Autodesk Inventor part; units mm, degrees
ref_plane "YZ Plane" through (0, 0, 0) normal (1, 0, 0) x (0, 1, 0)
ref_plane "XZ Plane" through (0, 0, 0) normal (0, 1, 0) x (-1, 0, 0)
ref_plane "XY Plane" through (0, 0, 0) normal (0, 0, 1) x (1, 0, 0)
sketch "Sketch1" plane through (0, 0, 0) normal (0, 0, 1) x (1, 0, 0)
  line L0 (0, 0) -> (9.525, 0)
  line L1 (9.525, 0) -> (9.525, 25.4)
  line L2 (9.525, 25.4) -> (0, 25.4)
  line L3 (0, 25.4) -> (0, 0)
  dimension "d0" = 9.525
  dimension "d1" = 25.4
extrude "Extrusion1" add sketch "Sketch1" along normal blind 95.25
sketch "Sketch2" plane through (0, 25.4, 0) normal (0, 1, 0) x (1, 0, 0)
  line L0 (0, 0) -> (0, -95.25) construction
  line L1 (0, -47.625) -> (9.525, -47.625) construction
  line L2 (9.525, 0) -> (9.525, -95.25) construction
  point P0 (4.7625, -19.05)
  point P1 (4.7625, -76.2)
  dimension "d4" = 19.05
  dimension "d5" = 4.7625
hole "Hole1" at (4.7625, 25.4, 19.05) at (4.7625, 25.4, 76.2) direction (0, -1, 0) diameter 2.6416 end through all
sketch "Sketch3" plane through (0, 0, 0) normal (-1, 0, 0) x (0, 0, 1)
  line L0 (0, 25.4) -> (0, 0) construction
  line L1 (0, 0) -> (95.25, 0) construction
  line L2 (95.25, 25.4) -> (95.25, 0) construction
  line L3 (0, 25.4) -> (95.25, 25.4) construction
  line L4 (7.9375, 19.8438) -> (11.1125, 19.8438)
  line L5 (11.1125, 19.8438) -> (11.1125, 15.0812)
  line L6 (11.1125, 15.0812) -> (7.9375, 15.0812)
  line L7 (7.9375, 15.0812) -> (7.9375, 19.8438)
  line L8 (7.9375, 19.8438) -> (11.1125, 15.0812) construction
  line L9 (11.1125, 19.8438) -> (7.9375, 15.0812) construction
  line L10 (0, 0) -> (95.25, 0) construction
  line L11 (47.625, 0) -> (47.625, 25.4) construction
  line L12 (87.3125, 19.8438) -> (84.1375, 19.8438)
  line L13 (84.1375, 19.8438) -> (84.1375, 15.0813)
  line L14 (84.1375, 15.0813) -> (87.3125, 15.0813)
  line L15 (87.3125, 15.0813) -> (87.3125, 19.8438)
  line L16 (87.3125, 19.8438) -> (84.1375, 15.0813) construction
  line L17 (84.1375, 19.8438) -> (87.3125, 15.0813) construction
  point P0 (9.525, 17.4625)
  point P1 (85.725, 17.4625)
  dimension "d13" = 3.175
  dimension "d14" = 4.7625
  dimension "d15" = 9.525
  dimension "d16" = 7.9375
extrude "Extrusion2" cut sketch "Sketch3" against normal through all
properties part number "ImagineFrameFront" material "Polycarbonate, Clear"
The listing builds one solid part. Answer for the finished solid, in the listing's coordinates (mm). A direction names the side the tool comes from. Round coordinates to 2 decimals unless told otherwise and drop trailing zeros. Write each loop counter-clockwise with the first axis right and the second up, starting at its lowest first coordinate (ties: lowest second). Pieces come first, ordered by that corner, then holes. Notation, with made-up numbers: (-26.5, -17) -> (9.5, -17) arc R13 ccw to (9.5, -9) -> close; hole circle Ø1 at (56.5, 47.25). An arc over 180 degrees is marked (long way). Use CSV: the item, a comma, the result in double quotes. Start each with the question number.
(1) Which of the six approach directions +Z, -Z, +X, -X, +Y, -Y give full straight-line access (tool end or side, diameter ignored) to faces 1 (the face through (9.525, 13, 47)), 2 (the face through (5, 15.081, 86))?
(2) Section A-A on z = 19.05 is taken. Give the vertices of the cut face in (x, y) (3 decimals), then the cut area to 3 significant figures.
(3) Consider L1, parallel to Z at x = 8.5, y = 16.5; L2, parallel to X at y = 12.5, z = 19.05 (3 decimals); L3, parallel to Y at x = 2.75, z = 8. Determine where each line is inside the solid, lowest interval first. Write a range as from..to.
(4) The mould has two halves that part along Z. Classify faces 3 (the face through (5, 13, 0)), 4 (the face through (5.27, 12.52, 77.42)), 5 (the face through (0, 13, 47)): released by +Z, released by -Z, zero draft, split by the parting line, or undercut.
A:
1,face 1,"+Z, -Z, +X, +Y, -Y"
1,face 2,"+X, -X"
2,outline,"(0, 0) -> (3.442, 0) -> (3.442, 25.4) -> (0, 25.4) -> close; (6.083, 0) -> (9.525, 0) -> (9.525, 25.4) -> (6.083, 25.4) -> close"
2,area,"175 mm²"
3,L1,"z = 0..7.94, 11.11..84.14, 87.31..95.25"
3,L2,"x = 0..3.442, 6.083..9.525"
3,L3,"y = 0..15.08, 19.84..25.4"
4,face 3,"released by -Z"
4,face 4,"undercut"
4,face 5,"zero draft"
